```python
from build123d import *

# Parameters (mm, degrees)
F0_W     = 15
F0_H     = 15
F1_DEPTH = 7.5
F2_R     = 4
F3_DEPTH = 5.5
F4_R     = 4
F5_DEPTH = 5.5
F6_R     = 3
F7_DEPTH = 15.001
F8_W     = 1
F8_H     = 1
F10_W    = 1
F10_H    = 1
F12_SIZE = 0.5
F13_R    = 2
F14_SIZE = 0.5


with BuildPart() as f1:
    # F0 (on Front) → F1 (new body, symmetric)
    with BuildSketch(Plane.XZ):
        Rectangle(F0_W, F0_H)
    extrude(amount=F1_DEPTH, both=True)

    # F2 (on face) → F3 (join)
    with BuildSketch(Plane.YZ.offset(7.5)):
        Circle(F2_R)
    extrude(amount=F3_DEPTH)

    # F4 (on face) → F5 (join)
    with BuildSketch(Plane(origin=(-7.5, 0, 0), x_dir=(0, -1, 0), z_dir=(-1, 0, 0))):
        Circle(F4_R)
    extrude(amount=F5_DEPTH)

    # F6 (on face) → F7 (cut, through all)
    with BuildSketch(Plane.XY.offset(7.5)):
        Circle(F6_R)
    extrude(amount=-F7_DEPTH, mode=Mode.SUBTRACT)

    # F8 (on Front) → F9 (revolve, cut)
    with BuildSketch(Plane.XZ):
        with Locations((10.5, 3.5)):
            Rectangle(F8_W, F8_H)
    revolve(axis=Axis((13, 0, 0), (1, 0, 0)), mode=Mode.SUBTRACT)

    # F10 (on Front) → F11 (revolve, cut)
    with BuildSketch(Plane.XZ):
        with Locations((-10.5, 3.5)):
            Rectangle(F10_W, F10_H)
    revolve(axis=Axis((-13, 0, 0), (-1, 0, 0)), mode=Mode.SUBTRACT)

    # F12
    f12_edges = [f1.edges().sort_by_distance(p)[0] for p in [
        (13, -4, 0),
        (-13, 4, 0),
    ]]
    chamfer(f12_edges, length=F12_SIZE)

    # F13
    f13_edges = [f1.edges().sort_by_distance(p)[0] for p in [
        (-7.5, -7.5, 0),
        (-7.5, 7.5, 0),
        (7.5, 7.5, 0),
        (7.5, -7.5, 0),
    ]]
    fillet(f13_edges, radius=F13_R)

    # F14
    f14_edges = [f1.edges().sort_by_distance(p)[0] for p in [
        (-3, 0, 7.5),
        (-3, 0, -7.5),
    ]]
    chamfer(f14_edges, length=F14_SIZE)


solid = f1.part
```
Source: CAD feature listing. Evaluate the final solid. Frame: model axes, mm. A direction names the side the tool comes from. Give positions to 0.01 mm unless a question says otherwise; leave off trailing zeros. Loops run counter-clockwise (first coordinate to the right, second up) from the corner with the lowest first, then second, coordinate; pieces in that order, holes last. Notation, with made-up numbers: M 54.25,55 L 93.25,55 A28 ccw 93.25,75 Z; hole C 22,-7 d10. An arc over 180 degrees is marked long. Put each result on its own line as item: value.
Q1. Mould query, pull axis X, two halves, no side actions, for faces 1 (the flat face through (-13, 0, 0)), 2 (the cylindrical face through (-8.732, -3.815, 1.201)), 3 (the flat face through (10, -3, -1)). Classes: released by +X, released by -X, zero draft, split by the parting line, or undercut.
Response values:
face 1: released by -X
face 2: zero draft
face 3: undercut
Q2. Pin query (flat end, axial travel): P1, Ø5, axis at y = 5, z = 1.5, coming from the +X side; P2, Ø3, axis at y = 4, z = -4, coming from the -X side. Return the tip coordinate at first contact, or that it passes through.
Response values:
P1: stops at x = 13
P2: stops at x = -7.5
Q3. Reachability of faces 4 (the flat face through (11, -3, -1)), 5 (the flat face through (0, -7.5, 0)), 6 (the cylindrical face through (11.74, 3.815, 1.201)), 7 (the flat face through (13, 0, 0)), 8 (the flat face through (-7.5, -4, -2)) from +Z, -Z, +X, -X, +Y, -Y: full face, straight path, thin tool, end or side. Return the list, or none.
Response values:
face 4: none
face 5: +Z, -Z, +X, -X, -Y
face 6: +X
face 7: +Z, -Z, +X, +Y, -Y
face 8: -X
Q4. Line query: probe 1 along Y at (x, z) = (0, -0.25); probe 2 along X at (y, z) = (0.5, -3.5); probe 3 along X at (y, z) = (3.75, 1). Output: solid intervals per line, ascending. Write a range as [from, to].
Response values:
probe 1: y = [-7.5, -3], [3, 7.5]
probe 2: x = [-12.96, -11], [-10, -2.96], [2.96, 10], [11, 12.96]
probe 3: x = [-12.62, -11], [-10, 10], [11, 12.62]
Q5. Section B-B (x = 0). Return the cut outline in (y, z).
Response values:
outline: M -7.5,-7.5 L -3.5,-7.5 L -3,-7 L -3,7 L -3.5,7.5 L -7.5,7.5 Z; M 3,-7 L 3.5,-7.5 L 7.5,-7.5 L 7.5,7.5 L 3.5,7.5 L 3,7 Z
Q6. Section C-C (y = 4.5). Return the cut outline in (x, z), and give its area (3 significant figures).
Response values:
outline: M -7.5,-7.5 L 7.5,-7.5 L 7.5,7.5 L -7.5,7.5 Z
area: 225 mm²
Q7. Section A-A (z = 5.25). Return the cut outline in (x, y), and give its area (3 significant figures).
Response values:
outline: M -7.5,-5.5 A2 ccw -5.5,-7.5 L 5.5,-7.5 A2 ccw 7.5,-5.5 L 7.5,5.5 A2 ccw 5.5,7.5 L -5.5,7.5 A2 ccw -7.5,5.5 Z; hole C 0,0 d6
area: 193 mm²
